The figure shows three views and two pictorial views of one solid part (mm, origin at its lowest corner). Answer the questions. A direction names the side the tool comes from. Coordinates: 2 decimals unless noted, no trailing zeros. Order: outer loops, then holes, each group sorted by start corner. A loop starts at its lowest first (then second) coordinate and runs counter-clockwise, first axis right, second up.
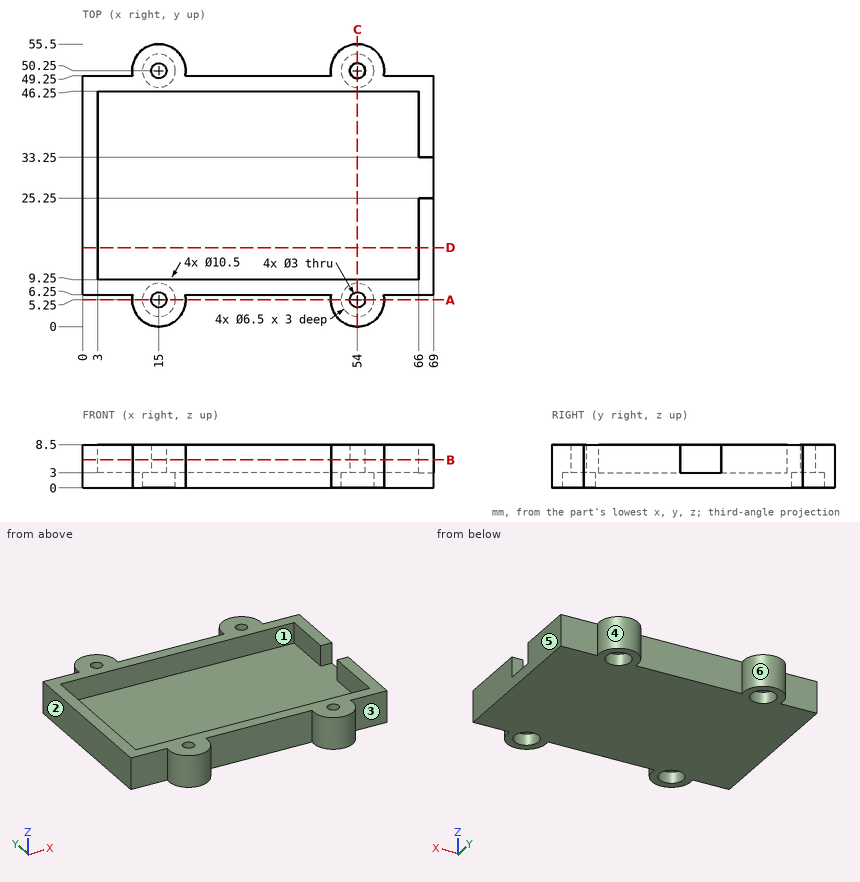
1) Each of these flat-tipped pins is pushed along its axis until it touches: P1, Ø2.5, axis at x = 67.5, z = 4.5, coming from the -Y side; P2, Ø3, axis at x = 36, z = 7, coming from the +Y side; P3, Ø5, axis at x = 49, z = 6.5, coming from the +Y side; P4, Ø2.5, axis at x = 54, y = 50.25, coming from the -Z side. Where does it stop, or does it pass through?
2) A cutting plane is placed at A-A, the plane y = 5.25. Write down the section's boundary in (x, z).
3) A cutting plane is placed at D-D, the plane y = 15.5. Write down the section's boundary in (x, z).
4) The mould has two halves that part along X. Classify the marked faces 3, 4, 5 and 6: released by +X, released by -X, zero draft, split by the parting line, or undercut.
5) Straight lines are drawn through the part: probe 1 along Y at (x, z) = (15, 5.7); probe 2 along Y at (x, z) = (54, 2.3); probe 3 along X at (y, z) = (21.5, 4.5). For each, find the intervals that lie inside material, in ascending order.
6) For the marked faces 1 and 2, determine the directions among +Z, -Z, +X, -X, +Y, -Y from which every point of the face is accessible in a straight line to the end or side of a thin tool.
7) A cutting plane is placed at C-C, the plane x = 54. Write down the section's boundary in (y, z), plus the area to 3 significant figures.
8) A cutting plane is placed at B-B, the plane z = 5.5. Write down the section's boundary in (x, y).
Working result:
1. P1: stops at y = 6.25
1. P2: stops at y = 49.25
1. P3: stops at y = 54.87
1. P4: passes through
2. outline: (9.75, 0) - (11.75, 0) - (11.75, 3) - (13.5, 3) - (13.5, 8.5) - (9.75, 8.5) - close; (16.5, 3) - (18.25, 3) - (18.25, 0) - (20.25, 0) - (20.25, 8.5) - (16.5, 8.5) - close; (48.75, 0) - (50.75, 0) - (50.75, 3) - (52.5, 3) - (52.5, 8.5) - (48.75, 8.5) - close; (55.5, 3) - (57.25, 3) - (57.25, 0) - (59.25, 0) - (59.25, 8.5) - (55.5, 8.5) - close
3. outline: (0, 0) - (69, 0) - (69, 8.5) - (66, 8.5) - (66, 3) - (3, 3) - (3, 8.5) - (0, 8.5) - close
4. face 3: zero draft
4. face 4: undercut
4. face 5: released by +X
4. face 6: undercut
5. probe 1: y = 0 to 3.75, 6.75 to 9.25, 46.25 to 48.75, 51.75 to 55.5
5. probe 2: y = 0 to 2, 8.5 to 47, 53.5 to 55.5
5. probe 3: x = 0 to 3, 66 to 69
6. face 1: +Z
6. face 2: +Z, -Z, -X, +Y, -Y
7. outline: (0, 0) - (2, 0) - (2, 3) - (3.75, 3) - (3.75, 8.5) - (0, 8.5) - close; (6.75, 3) - (8.5, 3) - (8.5, 0) - (47, 0) - (47, 3) - (48.75, 3) - (48.75, 8.5) - (46.25, 8.5) - (46.25, 3) - (9.25, 3) - (9.25, 8.5) - (6.75, 8.5) - close; (51.75, 3) - (53.5, 3) - (53.5, 0) - (55.5, 0) - (55.5, 8.5) - (51.75, 8.5) - close
7. area: 196 mm2
8. outline: (0, 6.25) - (9.85, 6.25) arc R5.25 ccw (long way) to (20.15, 6.25) - (48.85, 6.25) arc R5.25 ccw (long way) to (59.15, 6.25) - (69, 6.25) - (69, 25.25) - (66, 25.25) - (66, 9.25) - (3, 9.25) - (3, 46.25) - (66, 46.25) - (66, 33.25) - (69, 33.25) - (69, 49.25) - (59.15, 49.25) arc R5.25 ccw (long way) to (48.85, 49.25) - (20.15, 49.25) arc R5.25 ccw (long way) to (9.85, 49.25) - (0, 49.25) - close; hole circle Ø3 at (15, 5.25); hole circle Ø3 at (15, 50.25); hole circle Ø3 at (54, 5.25); hole circle Ø3 at (54, 50.25)
